Geometry check sheet. Reference: the model listing, model coordinates, mm. A direction names the side the tool comes from. Round coordinates to 2 decimals unless told otherwise and drop trailing zeros. Loops run counter-clockwise (first coordinate to the right, second up) from the corner with the lowest first, then second, coordinate; pieces in that order, holes last. Notation, with made-up numbers: (54.5, 83.5) -> (81.5, 83.5) arc R25 cw to (81.5, 120.5) -> close; hole circle Ø11 at (-17, 32). An arc over 180 degrees is marked (long way). Use a Markdown table: item, result. Add a question column.
Q1. Sectioned sample at A-A, the plane y = 35. Enter the section's corners in (x, z), then the cut area to 3 significant figures.
Q2. Release check for a two-part mould opening along X. For faces 3 (the face through (-70, 0, 51)), 4 (the face through (69, 0, 49)), 5 (the face through (-1, -50, 49)) record: released by +X, released by -X, zero draft, split by the parting line, or undercut.
Q3. Material ranges on L1, parallel to Z at x = 25, y = 31; L2, parallel to X at y = -7, z = 77; L3, parallel to Y at x = -37.5, z = 52, recorded low to high.
Q4. Sectioned sample at B-B, the plane x = 7.5. Enter the section's corners in (y, z).
Q5. Set-up check for faces 1 (the face through (-1, 0, 0)), 2 (the face through (-69, 0, 49)): record each of +Z, -Z, +X, -X, +Y, -Y from which the full face is reachable in a straight line by a thin tool's end or side.
```python
from build123d import *

# Parameters (mm, degrees)
SKETCH1_W           = 140
SKETCH1_H           = 100
BOSS_EXTRUDE1_DEPTH = 100
SHELL1_T            = -1
SKETCH2_W           = 140
SKETCH2_H           = 100
BOSS_EXTRUDE2_DEPTH = 1


with BuildPart() as part:
    # Sketch1 → Boss-Extrude1 (new body)
    with BuildSketch(Plane.XY):
        Rectangle(SKETCH1_W, SKETCH1_H)
    extrude(amount=BOSS_EXTRUDE1_DEPTH)

    # Shell1
    shell1_openings = [part.faces().sort_by_distance(p)[0] for p in [
        (0, 50, 50),
    ]]
    offset(amount=SHELL1_T, openings=shell1_openings, kind=Kind.INTERSECTION)

    # Sketch2 → Boss-Extrude2 (add)
    with BuildSketch(Plane(origin=(0, 50, 0), x_dir=(1, 0, 0), z_dir=(0, 1, 0))):
        with Locations((0, -50)):
            Rectangle(SKETCH2_W, SKETCH2_H)
    extrude(amount=BOSS_EXTRUDE2_DEPTH)


solid = part.part
```
Values:
| question | item | result |
|---|---|---|
| 1 | outline | (-70, 0) -> (70, 0) -> (70, 100) -> (-70, 100) -> close; hole (-69, 1) -> (69, 1) -> (69, 99) -> (-69, 99) -> close |
| 1 | area | 476 mm^2 |
| 2 | face 3 | released by -X |
| 2 | face 4 | undercut |
| 2 | face 5 | zero draft |
| 3 | L1 | 0 to 1, 99 to 100 |
| 3 | L2 | -70 to -69, 69 to 70 |
| 3 | L3 | -50 to -49, 50 to 51 |
| 4 | outline | (-50, 0) -> (51, 0) -> (51, 100) -> (-50, 100) -> close; hole (-49, 1) -> (50, 1) -> (50, 99) -> (-49, 99) -> close |
| 5 | face 1 | -Z, +X, -X, +Y, -Y |
| 5 | face 2 | none |
